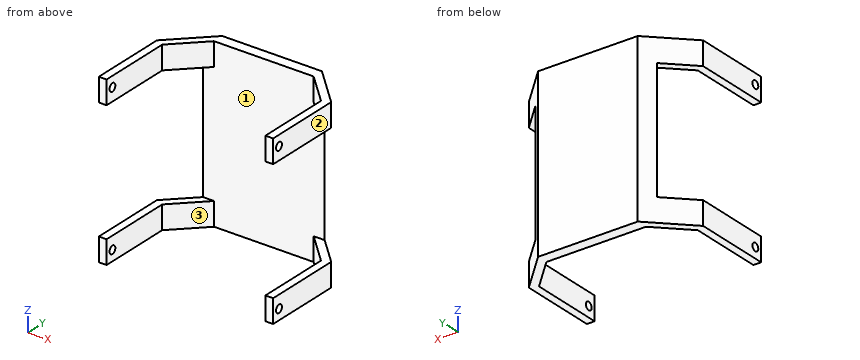
Autodesk Inventor part; units mm, degrees
ref_plane "YZ Plane" through (0, 0, 0) normal (1, 0, 0) x (0, 1, 0)
ref_plane "XZ Plane" through (0, 0, 0) normal (0, 1, 0) x (-1, 0, 0)
ref_plane "XY Plane" through (0, 0, 0) normal (0, 0, 1) x (1, 0, 0)
sketch "Sketch1" plane through (0, 0, 0) normal (1, 0, 0) x (0, 1, 0)
  line L0 (0, 0) -> (46.736, 0)
  line L1 (46.736, 0) -> (46.736, -68.58)
  line L2 (46.736, -68.58) -> (0, -68.58)
  line L3 (0, -68.58) -> (0, 0)
  dimension "d0" = 46.736
  dimension "d1" = 68.58
extrude "Extrusion1" add sketch "Sketch1" along normal blind 71.12
chamfer "Chamfer1" distance 15.24 angle 45 2 edges at (0, 46.736, -34.29) (71.12, 46.736, -34.29)
sketch "Sketch2" plane through (0, 0, 0) normal (0, 0, 1) x (1, 0, 0)
  line L0 (55.88, 46.736) -> (71.12, 31.496)
  line L1 (15.24, 46.736) -> (55.88, 46.736)
  line L2 (0, 31.496) -> (15.24, 46.736)
  line L3 (0, 0) -> (0, 31.496)
  line L4 (0, 0) -> (71.12, 0)
  line L5 (71.12, 31.496) -> (71.12, 0)
  line L6 (0, 0) -> (71.12, 0)
  line L7 (15.24, 42.2459) -> (55.88, 42.2459)
  line L8 (57.658, 0) -> (15.24, 0)
  line L9 (3.175, 0) -> (67.945, 0)
  line L10 (67.945, 0) -> (67.945, 30.1809)
  line L11 (3.175, 30.1809) -> (3.175, 0)
  line L12 (3.175, 30.1809) -> (15.24, 42.2459)
  line L13 (55.88, 42.2459) -> (67.945, 30.1809)
  dimension "d12" = 3.175
  dimension "d13" = 3.175
  dimension "d36" = 3.175
  dimension "d37" = 3.175
  dimension "d38" = 3.175
  dimension "d39" = 3.175
extrude "Extrusion2" cut sketch "Sketch2" against normal blind 127 contours L4 L11 L12 L7 L13 L10
sketch "Sketch3" plane through (71.12, 0, 0) normal (1, 0, 0) x (0, 0, -1)
  line L0 (0, 31.496) -> (68.58, 31.496)
  line L1 (0, 31.496) -> (0, 0)
  line L2 (0, 0) -> (68.58, 0)
  line L3 (68.58, 0) -> (68.58, 31.496)
  line L4 (4.2672, 3.175) -> (64.3128, 3.175)
  line L5 (64.3128, 3.175) -> (64.3128, 19.177)
  line L6 (64.3128, 19.177) -> (4.2672, 19.177)
  line L7 (4.2672, 19.177) -> (4.2672, 3.175)
  dimension "d16" = 60.0456
  dimension "d17" = 68.58
  dimension "d18" = 4.2672
  dimension "d19" = 16.002
  dimension "d20" = 31.496
  dimension "d21" = 3.175
hole "Hole2" at (71.12, 3.175, -4.2672) at (71.12, 3.175, -64.3128) direction (-1, 0, 0) diameter 3.175 end through all
sketch "Sketch4" plane through (71.12, 0, 0) normal (1, 0, 0) x (0, 0, -1)
  circle A0 centre (4.2672, 3.175) radius 1.5875
  circle A1 centre (64.3128, 3.175) radius 1.5875
  line L0 (0, 31.496) -> (68.58, 31.496)
  line L1 (0, 31.496) -> (0, 0)
  line L2 (0, 0) -> (68.58, 0)
  line L3 (68.58, 0) -> (68.58, 31.496)
  line L4 (0, 46.736) -> (0, 31.496)
  line L5 (0, 31.496) -> (68.58, 31.496)
  line L6 (68.58, 31.496) -> (68.58, 46.736)
  line L7 (68.58, 46.736) -> (0, 46.736)
  line L8 (68.58, 0) -> (0, 0)
  line L9 (0, 42.2459) -> (68.58, 42.2459)
  line L10 (9.525, 0) -> (59.055, 0)
  line L11 (59.055, 0) -> (59.055, 42.2459)
  line L12 (59.055, 42.2459) -> (9.525, 42.2459)
  line L13 (9.525, 42.2459) -> (9.525, 0)
  dimension "d40" = 42.2459
  dimension "d41" = 68.58
  dimension "d42" = 49.53
  dimension "d43" = 9.525
extrude "Extrusion3" cut sketch "Sketch4" against normal blind 127 contours L13 L9 L11 L0 | L0 L11 L2 L13
equation "\"d18\" = -0.5 * d16 + 0.5 * d17"
equation "\"d43\" = -0.5 * d42 + 0.5 * d41"
properties part number "MotorProtector"
Read the model definition and answer for the solid it produces. Units are mm, in the model's axes. Face numbers are marked on the shaded views. A direction names the side the tool comes from. Coordinates: 2 decimals unless noted, no trailing zeros. Order: outer loops, then holes, each group sorted by start corner. A loop starts at its lowest first (then second) coordinate and runs counter-clockwise, first axis right, second up. Notation, with made-up numbers: (2.25, 60) - (9.25, 60) arc R18 ccw to (9.25, 90) - close; hole circle Ø2 at (17.5, 49.5). An arc over 180 degrees is marked (long way). Answer as a JSON object with one key per item and string values. Group by question number.
Item 1: A flat-ended cylindrical pin translates along its axis: P1, Ø10, axis at x = 59.5, z = -43, coming from the -Y side. Find the tip coordinate at first contact, or state that the pin passes through.
Item 2: Section D-D (z = -20) is taken. Give the vertices of the cut face in (x, y), plus the area to 3 significant figures.
Item 3: A tool of negligible diameter and unlimited length cuts with its end or side. For the marked faces 1, 2 and 3, from which of +Z, -Z, +X, -X, +Y, -Y can it reach the whole face along a straight path? Write none if from no direction.
Item 4: Section A-A (y = 23) is taken. Give the vertices of the cut face in (x, z) (3 decimals), plus the area to 3 significant figures.
Item 5: Section B-B (x = 62) is taken. Give the vertices of the cut face in (y, z) (3 decimals), plus the area to 3 significant figures.
Item 6: Section C-C (y = 39) is taken. Give the vertices of the cut face in (x, z) (3 decimals).
Item 7: Consider probe 1 along Y at (x, z) = (18, -25); probe 2 along X at (y, z) = (30.5, -3.5); probe 3 along Y at (x, z) = (11, -32.5). Determine where each line is inside the solid, lowest interval first. Write a range as from..to.
Results are:
{
 "1": {"P1": "stops at y = 42.25"},
 "2": {"outline": "(10.75, 42.25) - (60.37, 42.25) - (55.88, 46.74) - (15.24, 46.74) - close", "area": "203 mm^2"},
 "3": {"face 1": "-Y", "face 2": "+Z, -Z, +X, +Y, -Y", "face 3": "+Z, -Z, -Y"},
 "4": {"outline": "(0, -68.58) - (3.175, -68.58) - (3.175, -59.055) - (0, -59.055) - close; (0, -9.525) - (3.175, -9.525) - (3.175, 0) - (0, 0) - close; (67.945, -68.58) - (71.12, -68.58) - (71.12, -59.055) - (67.945, -59.055) - close; (67.945, -9.525) - (71.12, -9.525) - (71.12, 0) - (67.945, 0) - close", "area": "121 mm^2"},
 "5": {"outline": "(36.126, -68.58) - (40.616, -68.58) - (40.616, -59.055) - (36.126, -59.055) - close; (36.126, -9.525) - (40.616, -9.525) - (40.616, 0) - (36.126, 0) - close", "area": "85.5 mm^2"},
 "6": {"outline": "(7.504, -68.58) - (11.994, -68.58) - (11.994, -59.055) - (7.504, -59.055) - close; (7.504, -9.525) - (11.994, -9.525) - (11.994, 0) - (7.504, 0) - close; (59.126, -68.58) - (63.616, -68.58) - (63.616, -59.055) - (59.126, -59.055) - close; (59.126, -9.525) - (63.616, -9.525) - (63.616, 0) - (59.126, 0) - close"},
 "7": {"probe 1": "y = 42.25..46.74", "probe 2": "x = 0..3.49, 67.63..71.12", "probe 3": "y = 42.25..42.5"}
}
